Autodesk Inventor part; units mm, degrees
ref_plane "YZ Plane" through (0, 0, 0) normal (1, 0, 0) x (0, 1, 0)
ref_plane "XZ Plane" through (0, 0, 0) normal (0, 1, 0) x (-1, 0, 0)
ref_plane "XY Plane" through (0, 0, 0) normal (0, 0, 1) x (1, 0, 0)
sketch "Sketch1" plane through (0, 0, 0) normal (0, 1, 0) x (-1, 0, 0)
  line L0 (0, 0) -> (-40, 0)
  line L1 (-40, 0) -> (-40, -30)
  line L2 (-40, -30) -> (0, -30)
  line L3 (0, -30) -> (0, 0)
  dimension "d0" = 40
  dimension "d1" = 30
extrude "Extrusion1" add sketch "Sketch1" along normal blind 5
sketch "Sketch2" plane through (0, 0, 0) normal (0, 0, 1) x (1, 0, 0)
  line L0 (0, 0) -> (40, 0) construction
  line L1 (40, 0) -> (40, 5) construction
  line L2 (0, 5) -> (40, 5) construction
  line L3 (0, 0) -> (0, 5) construction
  line L4 (40, 0) -> (40, 5)
  line L5 (40, 5) -> (35, 5)
  line L6 (35, 5) -> (35, 2)
  line L7 (35, 2) -> (40, 2)
  line L8 (40, 2) -> (40, 5)
  dimension "d4" = 3
  dimension "d5" = 5
extrude "Extrusion2" add sketch "Sketch2" along normal blind 3
fillet "Fillet1" radius 2 4 edges at (0, 2.5, 0) (0, 2.5, -30) (40, 2.5, -30) (40, 1, 0)
fillet "Fillet2" radius 1 18 edges at (35, 5, 1.5) (35, 2, 1.5) (40, 2, -1) (39.4142, 5, -29.4142) (20, 5, -30) (0.5858, 5, -29.4142) (0, 5, -15) (0.5858, 5, -0.5858) (18.5, 5, 0) (40, 5, -12.5) (40, 0, -15) (39.4142, 0, -29.4142) (20, 0, -30) (0.5858, 0, -29.4142) (0, 0, -15) (0.5858, 0, -0.5858) (20, 0, 0) (39.4142, 0, -0.5858)
properties part number "BATTERY_1S_560MAH_AKYGA"
Here's how the part is built. I have some questions about the finished solid (model axes, mm). A direction names the side the tool comes from. Coordinates: 2 decimals unless noted, no trailing zeros. Order: outer loops, then holes, each group sorted by start corner. A loop starts at its lowest first (then second) coordinate and runs counter-clockwise, first axis right, second up. Notation, with made-up numbers: M 68.5,60.5 L 107.5,60.5 A26 cw 107.5,98.5 Z; hole C -32,20 d3. An arc over 180 degrees is marked long. Answer as CSV lines item,"result". Start each with the question number.
1. I want a section at A-A, the plane x = 29. Write out the boundary of the cut face in (y, z), and give its area (3 significant figures).
2. On a 3-axis mill with a long thin cutter (end or side, diameter ignored), from which of +Z, -Z, +X, -X, +Y, -Y can I reach the whole of each face in a straight line? I mean faces 1 (the cylindrical face through (35.301, 4.715, 1.472)), 2 (the cylindrical face through (0.6, 2.52, -29.43)), 3 (the flat face through (35, 3.5, 1.5)), 4 (the flat face through (0, 2, -15)), 5 (the cylindrical face through (39.6, 1.6, -0.8)). Say none if no direction works.
3. I need wall thicknesses on line 1 (Z direction, x = 19, y = 3.7); line 2 (X direction, y = 3.4, z = 1); line 3 (X direction, y = 4.1, z = -4). Which ranges of each line are inside material? Lowest first, please. Write a range as [from, to].
4. For pin 1 (2.5 mm diameter, centred on x = 20, y = 3, fed in from +Z); pin 2 (1.1 mm diameter, centred on y = 3.5, z = 1, fed in from -X); pin 3 (1.5 mm diameter, centred on x = 37, z = 1, fed in from -Y), each with a flat end and sliding along its axis, tell me the tip position at first contact or that it passes through.
Recorded:
1,outline,"M 0,-29 A1 ccw 1,-30 L 4,-30 A1 ccw 5,-29 L 5,-1 A1 ccw 4,0 L 1,0 A1 ccw 0,-1 Z"
1,area,"149 mm2"
2,face 1,"+Z, -X, +Y"
2,face 2,"-Z, -X, +Y, -Y"
2,face 3,"+Z, -X, +Y, -Y"
2,face 4,"+Z, -Z, -X, +Y, -Y"
2,face 5,"+Z, +X, -Y"
3,line 1,"z = [-30, 0]"
3,line 2,"x = [35, 40]"
3,line 3,"x = [0.01, 39.99]"
4,pin 1,"stops at z = 0"
4,pin 2,"stops at x = 35"
4,pin 3,"stops at y = 2"
